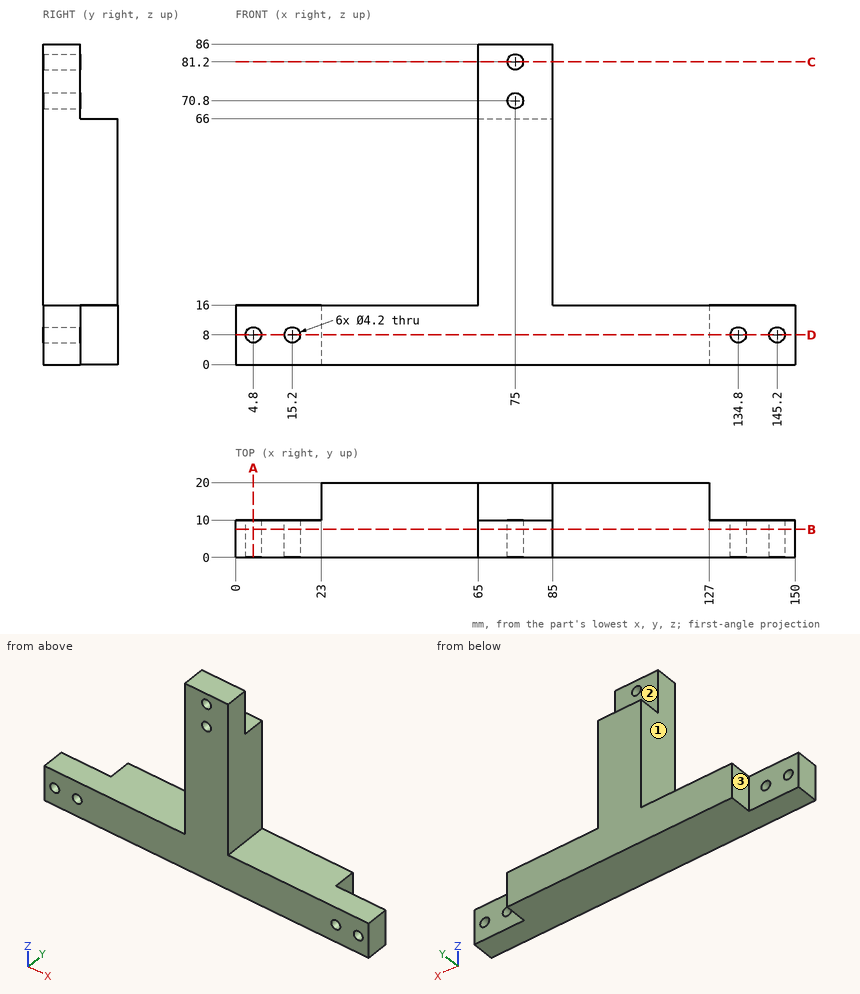
Drawing for the job (mm, zero at the part's lowest x, y, z). A direction names the side the tool comes from. Round coordinates to 2 decimals unless told otherwise and drop trailing zeros. Write each loop counter-clockwise with the first axis right and the second up, starting at its lowest first coordinate (ties: lowest second). Pieces come first, ordered by that corner, then holes. Notation, with made-up numbers: M 14.5,-0.75 L 57.5,-0.75 A29 ccw 57.5,22.25 Z; hole C 66,86.5 d1. An arc over 180 degrees is marked long. Put each result on its own line as item: value.
Item 1: Cut at B-B (y = 7.5). List the corners of the cut face in (x, z).
Responses:
outline: M 0,0 L 150,0 L 150,16 L 85,16 L 85,86 L 65,86 L 65,16 L 0,16 Z; hole C 4.8,8 d4.2; hole C 15.2,8 d4.2; hole C 75,70.8 d4.2; hole C 75,81.2 d4.2; hole C 134.8,8 d4.2; hole C 145.2,8 d4.2
Item 2: Cut at C-C (z = 81.2). List the corners of the cut face in (x, y).
Responses:
outline: M 65,0 L 72.9,0 L 72.9,10 L 65,10 Z; M 77.1,0 L 85,0 L 85,10 L 77.1,10 Z
Item 3: Cut at D-D (z = 8). List the corners of the cut face in (x, y), and give its area (3 significant figures).
Responses:
outline: M 0,0 L 2.7,0 L 2.7,10 L 0,10 Z; M 6.9,0 L 13.1,0 L 13.1,10 L 6.9,10 Z; M 17.3,0 L 132.7,0 L 132.7,10 L 127,10 L 127,20 L 23,20 L 23,10 L 17.3,10 Z; M 136.9,0 L 143.1,0 L 143.1,10 L 136.9,10 Z; M 147.3,0 L 150,0 L 150,10 L 147.3,10 Z
area: 2,370 mm²
Item 4: Probe L1, parallel to Z at x = 4.8, y = 6.25; L2, parallel to X at y = 6.25, z = 8; L3, parallel to X at y = 2.5, z = 8.5. List the from-to ranges inside material, lowest first. Write a range as from..to.
Responses:
L1: 0..5.9, 10.1..16
L2: 0..2.7, 6.9..13.1, 17.3..132.7, 136.9..143.1, 147.3..150
L3: 0..2.76, 6.84..13.16, 17.24..132.76, 136.84..143.16, 147.24..150
Item 5: Tool access for the marked faces 1, 2 and 3: list every direction of +Z, -Z, +X, -X, +Y, -Y with a clear straight run to the whole face (end or side of a thin tool).
Responses:
face 1: +Z, -X, +Y, -Y
face 2: +Z, +X, -X, +Y
face 3: +Z, -Z, -X, +Y
Item 6: Flat gauge pins, fed straight in: P1, Ø4, axis at x = 4.8, z = 8, coming from the -Y side; P2, Ø12, axis at x = 47.5, y = 9, coming from the +Z side; P3, Ø5, axis at x = 145.2, z = 8, coming from the +Y side; P4, Ø6, axis at y = 8, z = 68, coming from the -X side. Where does each tip first touch, or does it go through?
Responses:
P1: through
P2: z = 16
P3: y = 10
P4: x = 65
Item 7: Cut at A-A (x = 4.8). List the corners of the cut face in (y, z), and give its area (3 significant figures).
Responses:
outline: M 0,0 L 10,0 L 10,5.9 L 0,5.9 Z; M 0,10.1 L 10,10.1 L 10,16 L 0,16 Z
area: 118 mm²
